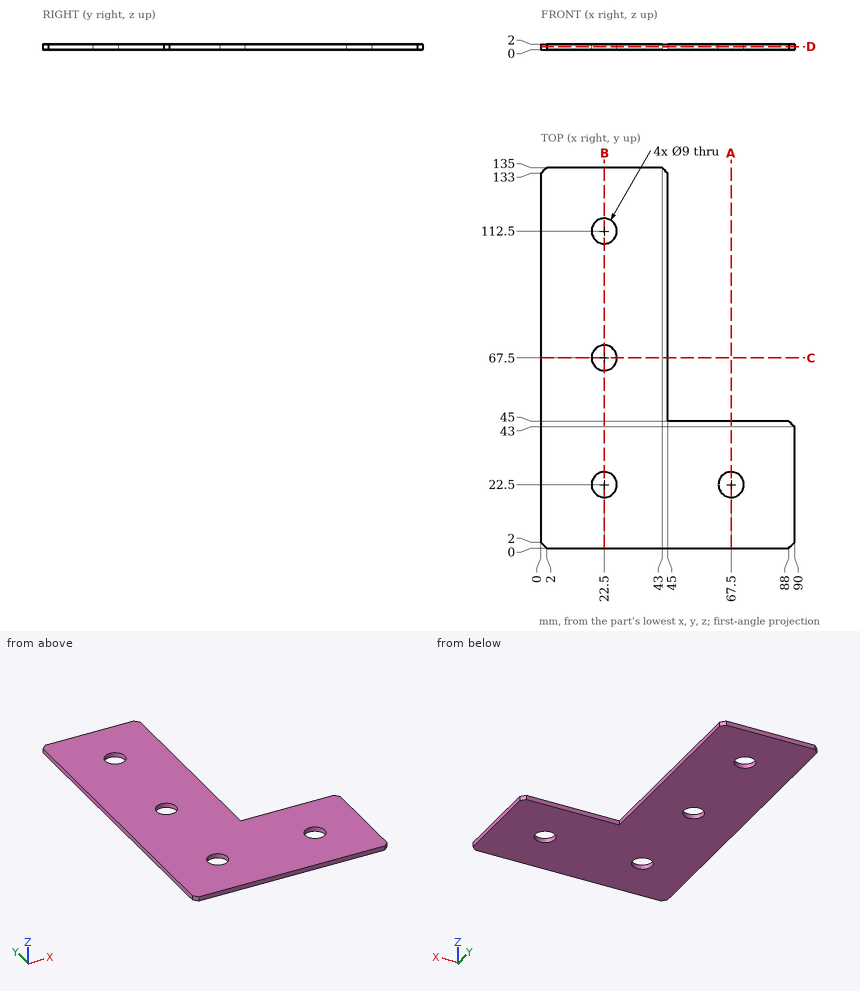
Answer from the drawing. Dimensions are ordinates in mm from the lowest x, y and z of the part. Coordinates: 2 decimals unless noted, no trailing zeros. Write each loop counter-clockwise with the first axis right and the second up, starting at its lowest first coordinate (ties: lowest second). Pieces come first, ordered by that corner, then holes. Notation, with made-up numbers: (83, 58.5) - (97, 58.5) arc R19 cw to (97, 68.5) - close; hole circle Ø9 at (-10.75, -1.5). An arc over 180 degrees is marked (long way). Return JSON: item names as keys, results as strings. Group by question number.
Q1. Flat-ended cylindrical pins translate along their axes: pin 1 Ø1 at (y, z) = (109.5, 0.5) entering from +X; pin 2 Ø1 at (x, z) = (56.5, 0.5) entering from +Y; pin 3 Ø7 at (x, y) = (22.5, 112.5) entering from -Z; pin 4 Ø14.5 at (x, y) = (22.5, 67.5) entering from -Z. Find the tip coordinate at first contact, or state that the pin passes through.
Q2. The part is cut by section A-A on x = 67.5. Write down the section's boundary in (y, z).
Q3. Find the intervals of material crossed by line 1 along X through (y, z) = (22.5, 1.25); line 2 along Y through (x, z) = (22.5, 0.5); line 3 along X through (y, z) = (67.5, 0.75), in increasing order. Write a range as [from, to].
Q4. The part is cut by section D-D on z = 1.05. Write down the section's boundary in (x, y).
Q5. The part is cut by section B-B on x = 22.5. Write down the section's boundary in (y, z), and give its area (3 significant figures).
Evaluation:
{
 "1": {"pin 1": "stops at x = 45", "pin 2": "stops at y = 45", "pin 3": "passes through", "pin 4": "stops at z = 0"},
 "2": {"outline": "(0, 0) - (18, 0) - (18, 2) - (0, 2) - close; (27, 0) - (45, 0) - (45, 2) - (27, 2) - close"},
 "3": {"line 1": "x = [0, 18], [27, 63], [72, 90]", "line 2": "y = [0, 18], [27, 63], [72, 108], [117, 135]", "line 3": "x = [0, 18], [27, 45]"},
 "4": {"outline": "(0, 2) - (2, 0) - (88, 0) - (90, 2) - (90, 43) - (88, 45) - (45, 45) - (45, 133) - (43, 135) - (2, 135) - (0, 133) - close; hole circle Ø9 at (22.5, 22.5); hole circle Ø9 at (22.5, 67.5); hole circle Ø9 at (22.5, 112.5); hole circle Ø9 at (67.5, 22.5)"},
 "5": {"outline": "(0, 0) - (18, 0) - (18, 2) - (0, 2) - close; (27, 0) - (63, 0) - (63, 2) - (27, 2) - close; (72, 0) - (108, 0) - (108, 2) - (72, 2) - close; (117, 0) - (135, 0) - (135, 2) - (117, 2) - close", "area": "216 mm2"}
}
